For this review, take the finished solid that the model builds, in its own axes (mm). Face numbers are marked on the shaded views. A direction names the side the tool comes from. Give positions to 0.01 mm unless a question says otherwise; leave off trailing zeros. Write each loop counter-clockwise with the first axis right and the second up, starting at its lowest first coordinate (ties: lowest second). Pieces come first, ordered by that corner, then holes.
from build123d import *

# Parameters (mm, degrees)
BOSS_EXTRUDE1_DEPTH = 42
SKETCH2_W           = 40
SKETCH2_H           = 7.5
BOSS_EXTRUDE2_DEPTH = 19
SKETCH3_W           = 19.7
SKETCH3_H           = 6
BOSS_EXTRUDE3_DEPTH = 40.45
RIB1_REACH          = 59.591
SKETCH4_WALL_W      = 159.669704532
SKETCH4_WALL_H      = 6
SKETCH7_R           = 1.7
CUT_EXTRUDE1_DEPTH  = 72.897792038


with BuildPart() as part:
    # Sketch1 → Boss-Extrude1 (new body)
    with BuildSketch(Plane.XY):
        Polygon((-3, -21.85), (-3, 21.85), (-20, 21.85), (-20, 24.85), (20, 24.85), (20, 21.85), (3, 21.85), (3, -21.85), (20, -21.85), (20, -24.85), (-20, -24.85), (-20, -21.85), align=None)
    extrude(amount=BOSS_EXTRUDE1_DEPTH)

    # Sketch2 → Boss-Extrude2 (add)
    with BuildSketch(Plane(origin=(0, -24.85, 0), x_dir=(-1, 0, 0), z_dir=(0, -1, 0))):
        with Locations((0, 3.75)):
            Rectangle(SKETCH2_W, SKETCH2_H)
    extrude(amount=-BOSS_EXTRUDE2_DEPTH)

    # Sketch3 → Boss-Extrude3 (add)
    with BuildSketch(Plane(origin=(0, 0, -7.5), x_dir=(-1, 0, 0), z_dir=(0, 0, -1))):
        with Locations((0, -8.85)):
            Rectangle(SKETCH3_W, SKETCH3_H)
    extrude(amount=BOSS_EXTRUDE3_DEPTH)

    # Sketch4 wall → Rib1 (add, up to next)
    with BuildSketch(Plane(origin=(0, -18.35, -27.725), x_dir=(0, -0.305971086836, 0.952040804809), z_dir=(0, -0.952040804809, -0.305971086836)), mode=Mode.PRIVATE) as rib1_sk1:
        Rectangle(SKETCH4_WALL_W, SKETCH4_WALL_H)
    rib1_tool1 = extrude(rib1_sk1.sketch, amount=-RIB1_REACH, mode=Mode.PRIVATE) - part.part
    add(rib1_tool1.solids().sort_by_distance((0, -18.35, -27.725))[0])

    # Sketch7 → Cut-Extrude1 (cut, through all)
    with BuildSketch(Plane.XZ.offset(24.85)):
        with Locations(Location((16, 30, 0), (0, 0, 270))):
            Circle(SKETCH7_R)
        with Locations(Location((16, 22, 0), (0, 0, 270))):
            Circle(SKETCH7_R)
        with Locations(Location((-16, 22, 0), (0, 0, 270))):
            Circle(SKETCH7_R)
        with Locations(Location((-16, 30, 0), (0, 0, 270))):
            Circle(SKETCH7_R)
    extrude(amount=-CUT_EXTRUDE1_DEPTH, mode=Mode.SUBTRACT)


solid = part.part
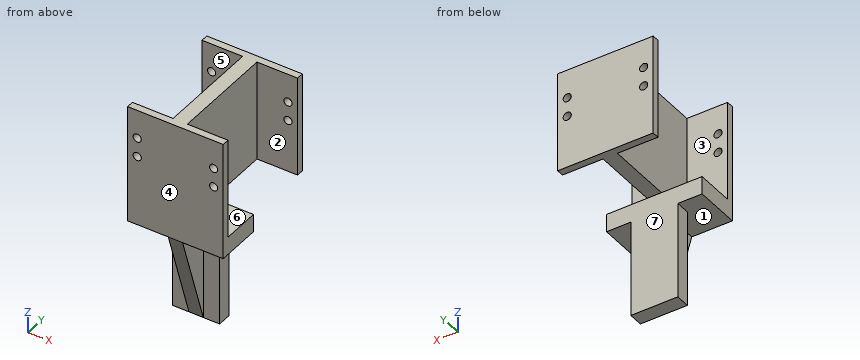
(1) We need section D-D (z = 4.5). Write out the cut boundary in (x, y), and give its area (3 significant figures).
(2) We need section B-B (x = 16). Write out the cut boundary in (y, z), and give its area (3 significant figures).
(3) We need section A-A (z = 30). Write out the cut boundary in (x, y).
(4) We need section C-C (x = 6.5). Write out the cut boundary in (y, z), and give its area (3 significant figures).
(5) The part is to be moulded in two halves that separate along Y. For the marked faces 1, 2, 3 and 4, say which applies: +Y half, -Y half, draft (parallel to the pull), parting line (faces both ways), or undercut.
(6) Clearance check with flat-ended pins moving along their axes: pin 1 Ø8 at (x, y) = (-6, 13.5) entering from -Z; pin 2 Ø8 at (x, y) = (12, -12.5) entering from +Z; pin 3 Ø1.5 at (y, z) = (17, 16.5) entering from -X. State where each tip first meets the part, or that it passes through.
(7) For L1, parallel to X at y = -24, z = 30; L2, parallel to Y at x = -10.5, z = 8.5; L3, parallel to X at y = 17.5, z = 38, list the stretches that pass through material, from the lowest coordinate up.
(8) Tool access review of the marked faces 5, 6 and 7: name each direction out of +Z, -Z, +X, -X, +Y, -Y from which nothing blocks a thin tool from reaching the whole face with its end or side.
The answers:
1. outline: (-20, -24.85) - (20, -24.85) - (20, -21.85) - (3, -21.85) - (3, 21.85) - (20, 21.85) - (20, 24.85) - (-20, 24.85) - (-20, 21.85) - (-3, 21.85) - (-3, -21.85) - (-20, -21.85) - close
1. area: 502 mm2
2. outline: (-24.85, -7.5) - (-5.85, -7.5) - (-5.85, 0) - (-21.85, 0) - (-21.85, 20.3) - (-24.85, 20.3) - close; (-24.85, 23.7) - (-21.85, 23.7) - (-21.85, 28.3) - (-24.85, 28.3) - close; (-24.85, 31.7) - (-21.85, 31.7) - (-21.85, 42) - (-24.85, 42) - close; (21.85, 0) - (24.85, 0) - (24.85, 20.3) - (21.85, 20.3) - close; (21.85, 23.7) - (24.85, 23.7) - (24.85, 28.3) - (21.85, 28.3) - close; (21.85, 31.7) - (24.85, 31.7) - (24.85, 42) - (21.85, 42) - close
2. area: 354 mm2
3. outline: (-20, -24.85) - (-17.7, -24.85) - (-17.7, -21.85) - (-20, -21.85) - close; (-20, 21.85) - (-17.7, 21.85) - (-17.7, 24.85) - (-20, 24.85) - close; (-14.3, -24.85) - (14.3, -24.85) - (14.3, -21.85) - (3, -21.85) - (3, 21.85) - (14.3, 21.85) - (14.3, 24.85) - (-14.3, 24.85) - (-14.3, 21.85) - (-3, 21.85) - (-3, -21.85) - (-14.3, -21.85) - close; (17.7, -24.85) - (20, -24.85) - (20, -21.85) - (17.7, -21.85) - close; (17.7, 21.85) - (20, 21.85) - (20, 24.85) - (17.7, 24.85) - close
4. outline: (-24.85, -7.5) - (-11.85, -7.5) - (-11.85, -47.95) - (-5.85, -47.95) - (-5.85, 0) - (-21.85, 0) - (-21.85, 42) - (-24.85, 42) - close; (21.85, 0) - (24.85, 0) - (24.85, 42) - (21.85, 42) - close
4. area: 637 mm2
5. face 1: draft
5. face 2: undercut
5. face 3: undercut
5. face 4: -Y half
6. pin 1: stops at z = 0
6. pin 2: stops at z = 0
6. pin 3: stops at x = -3
7. L1: x = -20 to -17.7, -14.3 to 14.3, 17.7 to 20
7. L2: y = -24.85 to -21.85, 21.85 to 24.85
7. L3: x = -3 to 3
8. face 5: +Z, -Z, -X
8. face 6: +Z, +X
8. face 7: -Z, +X, -X, +Y
